Autodesk Inventor part; units mm, degrees
ref_plane "YZ Plane" through (0, 0, 0) normal (1, 0, 0) x (0, 1, 0)
ref_plane "XZ Plane" through (0, 0, 0) normal (0, 1, 0) x (-1, 0, 0)
ref_plane "XY Plane" through (0, 0, 0) normal (0, 0, 1) x (1, 0, 0)
sketch "Sketch1" plane through (0, 0, 0) normal (0, 0, 1) x (1, 0, 0)
  line L0 (-20, 0) -> (20, 0)
  line L1 (20, 0) -> (20, -100)
  line L2 (20, -100) -> (-20, -100)
  line L3 (-20, -100) -> (-20, 0)
  point P0 (0, 0)
  point P1 (0, 0)
  dimension "d0" = 40
  dimension "d1" = 100
extrude "Plate1" add sketch "Sketch1" along normal blind 2
sketch "Sketch2" plane through (20, -100, 0) normal (1, 0, 0) x (0, 1, 0)
  line L0 (100, 0) -> (0, 0)
  line L1 (0, 0) -> (0, -33)
  line L2 (0, -33) -> (100, -33)
  line L3 (100, -33) -> (100, 0)
edge flange "Flange1" height 35 angle 90 thickness 2 bend radius 2.75 thickness toward (1, 0, 0) relief round relief width 2 relief depth 1 corner gap 2.75 corner form 0 edges at (20, -50, 0) (-20, -50, 0) wall of the first edge with corners at (20, 0, 0) (20, -100, 0) (20, -100, -33) (20, 0, -33)
bend "Bend1"
corner "Corner1"
sketch "Sketch5" plane through (-17.25, 0, 0) normal (0, 1, 0) x (1, 0, 0)
  line L0 (-4.75, 2.75) -> (-2.75, 2.75)
  line L1 (-2.75, 2.75) -> (-2.75, 33)
  line L2 (-2.75, 33) -> (-4.75, 33)
  line L3 (-4.75, 33) -> (-4.75, 2.75)
  line L4 (37.25, 2.75) -> (39.25, 2.75)
  line L5 (39.25, 2.75) -> (39.25, 33)
  line L6 (37.25, 33) -> (39.25, 33)
  line L7 (37.25, 2.75) -> (37.25, 33)
  point P0 (17.25, 0)
extrude "Extrusion2" add sketch "Sketch5" along normal blind 35
sketch "Sketch3" plane through (0, 0, 0) normal (1, 0, 0) x (0, 1, 0)
  line L0 (0, -33) -> (-100, -33)
  line L1 (-75, -20) -> (-75, -20) construction
  line L2 (-77.5, -20) -> (-77.5, -20)
  line L3 (-72.5, -20) -> (-72.5, -20)
  arc A0 (-72.5, -20) -> (-77.5, -20) centre (-75, -20) ccw
  arc A1 (-77.5, -20) -> (-72.5, -20) centre (-75, -20) ccw
  line L4 (-100, -2.75) -> (-100, -33)
  point P0 (0, 0)
  dimension "d14" = 0
  dimension "d15" = 13
  dimension "d17" = 2.5
  dimension "d18" = 25
extrude "Extrusion1" cut sketch "Sketch3" along normal through all both and the other way through all
pattern_linear "Rectangular Pattern1" count 3 spacing 50 along (0, 1, 0) of "Extrusion1"
fillet "Fillet1" radius 2 6 edges at (21, 35, -2.75) (-21, 35, -2.75) (-21, 35, -33) (21, 35, -33) (21, -100, -33) (-21, -100, -33)
equation "\"d2\" = Thickness"
equation "\"d3\" = BendReliefWidth"
equation "\"d4\" = BendReliefDepth"
equation "\"d5\" = MinimumRemnant"
equation "\"d6\" = TransitionRadius"
equation "\"d9\" = BendRadius"
equation "\"d10\" = CornerReliefSize"
equation "\"d11\" = GapSize"
equation "\"d12\" = JacobiRadiusSize"
equation "\"BendReliefWidth\" = Thickness"
equation "\"BendReliefDepth\" = 0.5 * Thickness"
equation "\"CornerReliefSize\" = 4 * Thickness"
equation "\"MinimumRemnant\" = 2 * Thickness"
equation "\"TransitionRadius\" = BendRadius"
equation "\"JacobiRadiusSize\" = BendRadius"
equation "\"GapSize\" = Thickness"
properties part number "NDM 4.0.8 bracket1" material "Stainless Steel"
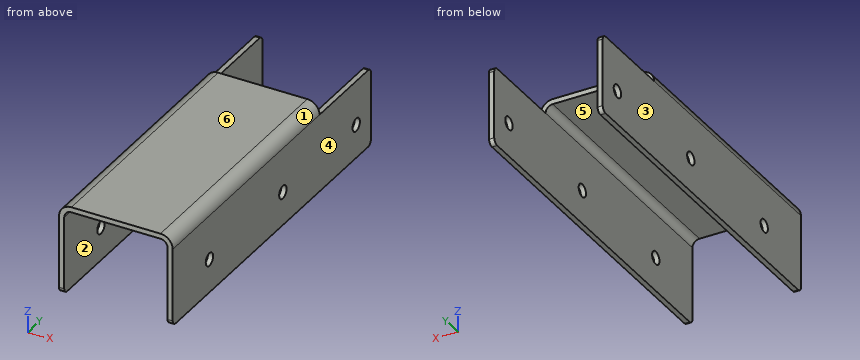
Can you work these out from the model? Positions are in its coordinate system, mm. Face numbers are marked on the shaded views. A direction names the side the tool comes from. Round coordinates to 2 decimals unless told otherwise and drop trailing zeros. Loops run counter-clockwise (first coordinate to the right, second up) from the corner with the lowest first, then second, coordinate; pieces in that order, holes last.
Item 1: If we mould it in two halves opening along X, with no side actions, what happens to the marked faces 3, 4, 5 and 6? For each: +X half, -X half, draft (parallel to the pull), parting line (faces both ways), or undercut.
Item 2: Suppose I cut it at D-D, the plane y = -75. Write out the boundary of the cut face in (x, z).
Item 3: Please list where these lines run through material, in increasing order: L1, parallel to X at y = -15.5, z = -4; L2, parallel to Z at x = -21, y = 25; L3, parallel to Z at x = -0.5, y = -64.
Item 4: Which directions (+Z, -Z, +X, -X, +Y, -Y) give clear straight access to the entire face, cutting with the end or side of a thin tool? Please do the marked faces 1 and 2.
Item 5: Suppose I cut it at A-A, the plane y = 11.5. Write out the boundary of the cut face in (x, z).
Item 6: Suppose I cut it at C-C, the plane y = 25. Write out the boundary of the cut face in (x, z).
Item 7: Suppose I cut it at B-B, the plane z = -10. Write out the boundary of the cut face in (x, y).
Item 8: Will these pins go through, and if not, where does the flat tip stop? pin 1 Ø2 at (y, z) = (-76.5, -1.5) entering from +X; pin 2 Ø4.5 at (y, z) = (25, -20) entering from +X; pin 3 Ø0.6 at (x, y) = (-20.5, 13) entering from +Z; pin 4 Ø1.4 at (x, z) = (-7, 0.5) entering from +Y.
Reported:
1. face 3: -X half
1. face 4: +X half
1. face 5: undercut
1. face 6: draft
2. outline: (-22, -33) - (-20, -33) - (-20, -22.5) - (-22, -22.5) - close; (-22, -17.5) - (-20, -17.5) - (-20, -2.75) arc R2.75 cw to (-17.25, 0) - (17.25, 0) arc R2.75 cw to (20, -2.75) - (20, -17.5) - (22, -17.5) - (22, -2.75) arc R4.75 ccw to (17.25, 2) - (-17.25, 2) arc R4.75 ccw to (-22, -2.75) - close; (20, -33) - (22, -33) - (22, -22.5) - (20, -22.5) - close
3. L1: x = -22 to -20, 20 to 22
3. L2: z = -33 to -22.5, -17.5 to -2.75
3. L3: z = 0 to 2
4. face 1: +Z, +X, +Y, -Y
4. face 2: -Z, +Y, -Y
5. outline: (-22, -33) - (-20, -33) - (-20, -2.75) - (-22, -2.75) - close; (20, -33) - (22, -33) - (22, -2.75) - (20, -2.75) - close
6. outline: (-22, -33) - (-20, -33) - (-20, -22.5) - (-22, -22.5) - close; (-22, -17.5) - (-20, -17.5) - (-20, -2.75) - (-22, -2.75) - close; (20, -33) - (22, -33) - (22, -22.5) - (20, -22.5) - close; (20, -17.5) - (22, -17.5) - (22, -2.75) - (20, -2.75) - close
7. outline: (-22, -100) - (-20, -100) - (-20, 35) - (-22, 35) - close; (20, -100) - (22, -100) - (22, 35) - (20, 35) - close
8. pin 1: stops at x = 21.99
8. pin 2: passes through
8. pin 3: stops at z = -2.75
8. pin 4: stops at y = 0
